from build123d import *

# Parameters (mm, degrees)
SKETCH1_W           = 7
SKETCH1_H           = 7
BOSS_EXTRUDE1_DEPTH = 15
SKETCH2_W           = 3.5
SKETCH2_H           = 3.5
BOSS_EXTRUDE2_DEPTH = 4
SKETCH3_W           = 3.5
SKETCH3_H           = 3.5
BOSS_EXTRUDE3_DEPTH = 4


with BuildPart() as part:
    # Sketch1 → Boss-Extrude1 (new, symmetric)
    with BuildSketch(Plane(origin=(0, 0, 0), x_dir=(1, 0, 0), z_dir=(0, 1, 0))):
        Rectangle(SKETCH1_W, SKETCH1_H)
    extrude(amount=BOSS_EXTRUDE1_DEPTH, both=True)

    # Sketch2 → Boss-Extrude2 (add)
    with BuildSketch(Plane(origin=(0, 15, 0), x_dir=(1, 0, 0), z_dir=(0, 1, 0))):
        Rectangle(SKETCH2_W, SKETCH2_H)
    extrude(amount=BOSS_EXTRUDE2_DEPTH)

    # Sketch3 → Boss-Extrude3 (add)
    with BuildSketch(Plane.XZ.offset(15)):
        Rectangle(SKETCH3_W, SKETCH3_H)
    extrude(amount=BOSS_EXTRUDE3_DEPTH)


solid = part.part
Model file for the job. Use its own axes, mm. A direction names the side the tool comes from. Round coordinates to 2 decimals unless told otherwise and drop trailing zeros. Order: outer loops, then holes, each group sorted by start corner. A loop starts at its lowest first (then second) coordinate and runs counter-clockwise, first axis right, second up.
(1) Drill centre lines: line 1 (Y direction, x = 3.25, z = 2.75); line 2 (X direction, y = 17, z = 1.5). Where is each one in solid material? Low to high.
(2) Band-saw the part on A-A (x = -0.75). List the corners of the cut face in (y, z), then the cut area to 3 significant figures.
(3) Band-saw the part on B-B (z = -0.25). List the corners of the cut face in (x, y).
(4) Band-saw the part on C-C (y = -15.5). List the corners of the cut face in (x, z), then the cut area to 4 significant figures.
(5) Pin check, flat tips, straight feed: pin 1 (1.8 mm diameter, centred on y = -16, z = -0.5, fed in from +X); pin 2 (1 mm diameter, centred on x = -0.5, y = -17, fed in from +Z); pin 3 (1.8 mm diameter, centred on x = 0, y = 17, fed in from -Z). Stop position of each tip, or through.
(6) 3-axis set-ups, long thin cutter, end or side, ignore diameter. For faces 1 (the face through (0, -17, -1.75)), 2 (the face through (-1.75, -17, 0)), 3 (the face through (0, 17, 1.75)), 4 (the face through (1.75, -17, 0)), 5 (the face through (0, -17, 1.75)): which of +Z, -Z, +X, -X, +Y, -Y reach the whole face in a straight line?
(7) Band-saw the part on D-D (x = 3). List the corners of the cut face in (y, z).
Verdict:
1. line 1: y = -15 to 15
1. line 2: x = -1.75 to 1.75
2. outline: (-19, -1.75) - (-15, -1.75) - (-15, -3.5) - (15, -3.5) - (15, -1.75) - (19, -1.75) - (19, 1.75) - (15, 1.75) - (15, 3.5) - (-15, 3.5) - (-15, 1.75) - (-19, 1.75) - close
2. area: 238 mm2
3. outline: (-3.5, -15) - (-1.75, -15) - (-1.75, -19) - (1.75, -19) - (1.75, -15) - (3.5, -15) - (3.5, 15) - (1.75, 15) - (1.75, 19) - (-1.75, 19) - (-1.75, 15) - (-3.5, 15) - close
4. outline: (-1.75, -1.75) - (1.75, -1.75) - (1.75, 1.75) - (-1.75, 1.75) - close
4. area: 12.25 mm2
5. pin 1: stops at x = 1.75
5. pin 2: stops at z = 1.75
5. pin 3: stops at z = -1.75
6. face 1: -Z, +X, -X, -Y
6. face 2: +Z, -Z, -X, -Y
6. face 3: +Z, +X, -X, +Y
6. face 4: +Z, -Z, +X, -Y
6. face 5: +Z, +X, -X, -Y
7. outline: (-15, -3.5) - (15, -3.5) - (15, 3.5) - (-15, 3.5) - close
